Here's how the part is built. I have some questions about the finished solid (model axes, mm). A direction names the side the tool comes from. Coordinates: 2 decimals unless noted, no trailing zeros. Order: outer loops, then holes, each group sorted by start corner. A loop starts at its lowest first (then second) coordinate and runs counter-clockwise, first axis right, second up. Notation, with made-up numbers: (16.25, 48.25) - (30.25, 48.25) arc R16 ccw to (30.25, 76.25) - close; hole circle Ø9 at (26.25, 72.25). An arc over 180 degrees is marked (long way). Answer as CSV lines item,"result". Start each with the question number.
Q1. I need wall thicknesses on line 1 (Y direction, x = 8.25, z = 25.5); line 2 (Z direction, x = 4.5, y = -10.5); line 3 (Z direction, x = -4.5, y = -15.25). Which ranges of each line are inside material? Lowest first, please.
Q2. Suppose I cut it at B-B (z = 12.5). Please give me the cut outline in (x, y), then the cut area to 3 significant figures.
Q3. For pin 1 Ø6 at (x, y) = (4, -14) entering from -Z; pin 2 Ø5 at (x, z) = (1.5, 13.5) entering from -Y, each with a flat end and sliding along its axis, tell me the tip position at first contact or that it passes through.
Q4. For faces 1 (the face through (-5.687, -3, 17)), 2 (the face through (-5.117, -14.437, 32.864)), 3 (the face through (3, -14, 32.263)), which set-ups out of +Z, -Z, +X, -X, +Y, -Y let a thin tool reach every point of the face, with its end or its side?
Q5. Suppose I cut it at C-C (x = 7.5). Please give me the cut outline in (y, z).
Q6. Suppose I cut it at A-A (y = -11.5). Please give me the cut outline in (x, z), then the cut area to 3 significant figures.
from build123d import *

# Parameters (mm, degrees)
F0_W     = 15
F0_H     = 15
F1_DEPTH = 35
F2_W     = 15
F2_H     = 2.73731336
F3_DEPTH = 10
F4_R     = 2
F5_R     = 2


with BuildPart() as f1:
    # F0 (on Top) → F1 (new body)
    with BuildSketch(Plane.XY):
        with Locations((1.8129660748, -1.8668582881)):
            Rectangle(F0_W, F0_H)
    extrude(amount=F1_DEPTH)

    # F2 (on face) → F3 (join)
    with BuildSketch(Plane.XZ.offset(9.3668582881)):
        with Locations((1.8129660748, 33.63134332)):
            Rectangle(F2_W, F2_H)
    extrude(amount=F3_DEPTH)

    # F4
    f4_edges = [f1.edges().sort_by_distance(p)[0] for p in [
        (-5.687034, 5.633142, 17.5),
    ]]
    fillet(f4_edges, radius=F4_R)

    # F5
    f5_edges = [f1.edges().sort_by_distance(p)[0] for p in [
        (-5.687034, -14.366858, 32.262687),
    ]]
    fillet(f5_edges, radius=F5_R)


solid = f1.part
Here are the results:
1,line 1,"y = -9.37 to 5.63"
1,line 2,"z = 32.26 to 35"
1,line 3,"z = 32.44 to 35"
2,outline,"(-5.69, -9.37) - (9.31, -9.37) - (9.31, 5.63) - (-3.69, 5.63) arc R2 ccw to (-5.69, 3.63) - close"
2,area,"224 mm²"
3,pin 1,"stops at z = 32.26"
3,pin 2,"stops at y = -9.37"
4,face 1,"+Z, -Z, -X, +Y, -Y"
4,face 2,"-Z, -X, -Y"
4,face 3,"-Z, +X, -X, -Y"
5,outline,"(-19.37, 32.26) - (-9.37, 32.26) - (-9.37, 0) - (5.63, 0) - (5.63, 35) - (-19.37, 35) - close"
6,outline,"(-5.69, 34.26) arc R2 ccw to (-3.69, 32.26) - (9.31, 32.26) - (9.31, 35) - (-5.69, 35) - close"
6,area,"40.2 mm²"
